```python
from build123d import *

# Parameters (mm, degrees)
EXTRUDE_1_DEPTH = 2
SKETCH_2_W      = 1
SKETCH_2_H      = 15
EXTRUDE_2_DEPTH = 8


with BuildPart() as part:
    # 草图1 → 凸台-拉伸1 (new body)
    with BuildSketch(Plane.XY):
        with BuildLine():
            Line((1.5, -13.673349455), (1.5, -29.673349455))
            ThreePointArc((1.5, -29.673349455), (0, -31.173349455), (-1.5, -29.673349455))
            Line((-1.5, -29.673349455), (-1.5, -13.673349455))
            ThreePointArc((-1.5, -13.673349455), (0, -12.173349455), (1.5, -13.673349455))
        make_face()
    extrude(amount=EXTRUDE_1_DEPTH)

    # 草图2 → 凸台-拉伸2 (add)
    with BuildSketch(Plane(origin=(0, 0, 0), x_dir=(-1, 0, 0), z_dir=(0, 0, -1))):
        with Locations((0.022272941, -21.592941234)):
            Rectangle(SKETCH_2_W, SKETCH_2_H)
    extrude(amount=EXTRUDE_2_DEPTH)


solid = part.part
```
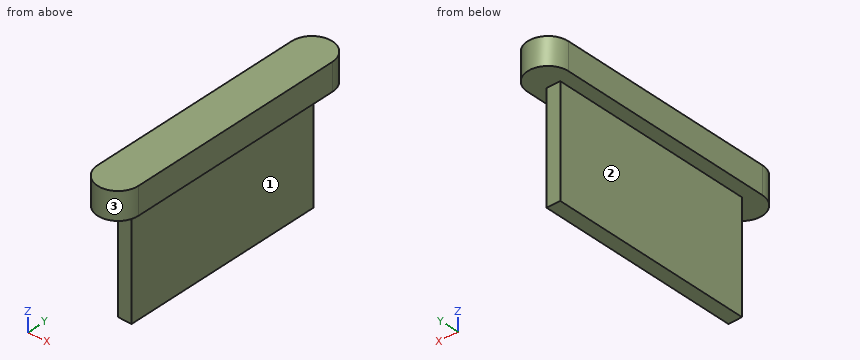
The model under review builds one solid part; all positions refer to its coordinate system, in mm. Face numbers are marked on the shaded views. A direction names the side the tool comes from. Round coordinates to 2 decimals unless told otherwise and drop trailing zeros. Loops run counter-clockwise (first coordinate to the right, second up) from the corner with the lowest first, then second, coordinate; pieces in that order, holes last. Notation, with made-up numbers: (-19.5, 53) -> (-13.5, 53) arc R22 cw to (-13.5, 89) -> close; hole circle Ø10 at (6.5, 46.25). An arc over 180 degrees is marked (long way). Answer as a JSON object with one key per item and string values. Group by question number.
1) We need section A-A on y = -15.75. Write out the cut boundary in (x, z), then the cut area to 3 significant figures.
2) We need section B-B on x = 0. Write out the cut boundary in (y, z).
3) We need section C-C on z = 1. Write out the cut boundary in (x, y), then the cut area to 3 significant figures.
4) For pin 1 Ø0.8 at (x, z) = (0, -2.5) entering from -Y; pin 2 Ø1 at (x, z) = (-0.5, -4) entering from +Y; pin 3 Ø2.5 at (y, z) = (-19, -5) entering from +X, all flat-tipped, find the tip position at first contact; note any pin that passes through.
5) For line 1 (Z direction, x = 1.25, y = -23.5); line 2 (X direction, y = -26.25, z = -5); line 3 (Y direction, x = 0.2, z = -7.5), list the stretches that pass through material, from the lowest coordinate up. Write a range as [from, to].
6) We need section D-D on z = -5. Write out the cut boundary in (x, y).
7) For the marked faces 1, 2 and 3, list the 3-axis set-ups (+Z, -Z, +X, -X, +Y, -Y) from which the entire face can be reached by the end or side of a thin tool; tool diameter is ignored.
Result set:
{
 "1": {"outline": "(-1.5, 0) -> (-0.52, 0) -> (-0.52, -8) -> (0.48, -8) -> (0.48, 0) -> (1.5, 0) -> (1.5, 2) -> (-1.5, 2) -> close", "area": "14.0 mm²"},
 "2": {"outline": "(-31.17, 0) -> (-29.09, 0) -> (-29.09, -8) -> (-14.09, -8) -> (-14.09, 0) -> (-12.17, 0) -> (-12.17, 2) -> (-31.17, 2) -> close"},
 "3": {"outline": "(-1.5, -29.67) arc R1.5 ccw to (1.5, -29.67) -> (1.5, -13.67) arc R1.5 ccw to (-1.5, -13.67) -> close", "area": "55.1 mm²"},
 "4": {"pin 1": "y = -29.09", "pin 2": "y = -14.09", "pin 3": "x = 0.48"},
 "5": {"line 1": "[0, 2]", "line 2": "[-0.52, 0.48]", "line 3": "[-29.09, -14.09]"},
 "6": {"outline": "(-0.52, -29.09) -> (0.48, -29.09) -> (0.48, -14.09) -> (-0.52, -14.09) -> close"},
 "7": {"face 1": "-Z, +X, +Y, -Y", "face 2": "-Z, -X, +Y, -Y", "face 3": "+Z, -Z, -Y"}
}
